Autodesk Inventor part; units mm, degrees
ref_plane "YZ Plane" through (0, 0, 0) normal (1, 0, 0) x (0, 1, 0)
ref_plane "XZ Plane" through (0, 0, 0) normal (0, 1, 0) x (-1, 0, 0)
ref_plane "XY Plane" through (0, 0, 0) normal (0, 0, 1) x (1, 0, 0)
sketch "Sketch1" plane through (0, 0, 0) normal (0, 1, 0) x (-1, 0, 0)
  line L0 (50, 37.5) -> (-50, 37.5)
  line L1 (-50, 37.5) -> (-50, -37.5)
  line L2 (-50, -37.5) -> (50, -37.5)
  line L3 (50, -37.5) -> (50, 37.5)
  line L4 (50, 37.5) -> (-50, -37.5) construction
  line L5 (-50, 37.5) -> (50, -37.5) construction
  line L6 (0, 0) -> (-10, 0)
  line L7 (-10, 0) -> (-10, 8)
  line L8 (-10, 0) -> (-2, 0) construction
  line L9 (-10, 0) -> (-10, -8)
  line L10 (-10, 0) -> (-2, 0) construction
  line L11 (-10, 8) -> (-43, 8) construction
  line L12 (-10, 9.6) -> (-43, 9.6)
  line L13 (-43, 6.4) -> (-10, 6.4)
  arc A0 (-10, 6.4) -> (-10, 9.6) centre (-10, 8) ccw
  arc A1 (-43, 9.6) -> (-43, 6.4) centre (-43, 8) ccw
  line L14 (-10, 8) -> (23, 8) construction
  line L15 (0, 0) -> (-50, 0)
  line L16 (-10, -8) -> (-43, -8) construction
  line L17 (-10, -6.4) -> (-43, -6.4)
  line L18 (-43, -9.6) -> (-10, -9.6)
  arc A2 (-10, -9.6) -> (-10, -6.4) centre (-10, -8) ccw
  arc A3 (-43, -6.4) -> (-43, -9.6) centre (-43, -8) ccw
  line L19 (-10, -8) -> (23, -8) construction
  line L20 (0, 37.5) -> (0, -37.5)
  line L21 (10, 0) -> (10, 8)
  line L22 (10, 0) -> (10, -8)
  line L23 (10, 8) -> (43, 8) construction
  line L24 (10, 9.6) -> (43, 9.6)
  line L25 (43, 6.4) -> (10, 6.4)
  arc A4 (10, 9.6) -> (10, 6.4) centre (10, 8) ccw
  arc A5 (43, 6.4) -> (43, 9.6) centre (43, 8) ccw
  line L26 (10, -8) -> (43, -8) construction
  line L27 (10, -6.4) -> (43, -6.4)
  line L28 (43, -9.6) -> (10, -9.6)
  arc A6 (10, -6.4) -> (10, -9.6) centre (10, -8) ccw
  arc A7 (43, -9.6) -> (43, -6.4) centre (43, -8) ccw
  point P0 (-26.5, 8)
  point P1 (-26.5, -8)
  point P2 (26.5, 8)
  point P3 (26.5, -8)
  dimension "d0" = 100
  dimension "d1" = 75
  dimension "d2" = 10
  dimension "d3" = 8
  dimension "d4" = 90
  dimension "d5" = 8
  dimension "d6" = 90
  dimension "d7" = 33
  dimension "d8" = 180
  dimension "d9" = 3.2
  dimension "d10" = 33
  dimension "d11" = 180
  dimension "d12" = 3.2
extrude "Extrusion1" add sketch "Sketch1" along normal blind 10
sketch "Sketch2" plane through (0, 10, 0) normal (0, 1, 0) x (1, 0, 0)
  line L0 (50, 37.5) -> (-50, 37.5)
  line L1 (-50, 37.5) -> (50, 37.5)
  line L2 (50, 37.5) -> (50, 84.5)
  line L3 (50, 84.5) -> (-50, 84.5)
  line L4 (-50, 84.5) -> (-50, 37.5)
  point P0 (0, 0)
  dimension "d15" = 47
extrude "Extrusion2" add sketch "Sketch2" against normal blind 10
sketch "Sketch3" plane through (0, 10, 0) normal (0, 1, 0) x (1, 0, 0)
  line L0 (38.0429, 35.7373) -> (1.3429, 35.7373)
  line L1 (1.3429, 35.7373) -> (1.3429, 72.4373)
  line L2 (1.3429, 72.4373) -> (38.0429, 72.4373)
  line L3 (38.0429, 72.4373) -> (38.0429, 35.7373)
  circle A0 centre (1.3429, 72.4373) radius 1.65
  circle A1 centre (1.3429, 35.7373) radius 1.65
  circle A2 centre (38.0429, 35.7373) radius 1.65
  circle A3 centre (38.0429, 72.4373) radius 1.65
  line L4 (-28.9751, 35.7373) -> (-28.9751, 72.4373)
  circle A4 centre (-28.9751, 72.4373) radius 1.65
  circle A5 centre (-28.9751, 35.7373) radius 1.65
  point P0 (0, 0)
  dimension "d18" = 36.7
  dimension "d19" = 36.7
  dimension "d20" = 3.3
  dimension "d21" = 3.3
  dimension "d22" = 3.3
  dimension "d23" = 3.3
  dimension "d24" = 36.7
  dimension "d25" = 3.3
  dimension "d26" = 3.3
extrude "Extrusion3" cut sketch "Sketch3" against normal blind 10 contours A1 L1 L0 | L0 L1 A1 | A2 L3 L0 | L0 L3 A2 | A0 L2 L1 | L1 L2 A0 | A3 L2 L3 | L3 L2 A3 | A4 | A5
sketch "Sketch4" plane through (0, 10, 0) normal (0, 1, 0) x (1, 0, 0)
  point P0 (0, 0)
fillet "Fillet1" radius 7 4 edges at (-50, 5, 37.5) (50, 5, 37.5) (50, 5, -84.5) (-50, 5, -84.5)
properties part number "bas" material "Polycarbonate, Clear"
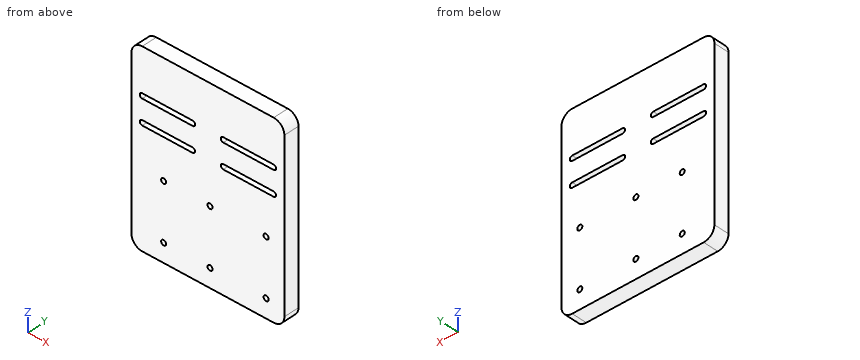
The listing builds one solid part. Answer for the finished solid, in the listing's coordinates (mm). Coordinates: 2 decimals unless noted, no trailing zeros. Loops run counter-clockwise (first coordinate to the right, second up) from the corner with the lowest first, then second, coordinate; pieces in that order, holes last. Notation, with made-up numbers: (-14.75, 0.25) - (36.25, 0.25) arc R24 cw to (36.25, 18.25) - close; hole circle Ø1 at (-32, -32). An arc over 180 degrees is marked (long way). Use a Markdown table: item, result. Add a question column.
1) The part is cut by section C-C, the plane y = 4. State how many separate pieces and enclosed holes the cut face has, and give its area (3 significant figures).
2) The part is cut by section B-B, the plane z = 8. Give the vertices of the cut face in (x, y).
3) Find the intervals of material crossed by line 1 (Z direction, x = -13, y = 5.75); line 2 (Z direction, x = -29, y = 8.75); line 3 (X direction, y = 4.25, z = -73.5), in increasing order.
4) The part is cut by section A-A, the plane x = -21. Give the vertices of the cut face in (y, z).
Here are the results:
| question | item | result |
|---|---|---|
| 1 | separate pieces | 1 |
| 1 | enclosed holes | 10 |
| 1 | area | 11,700 mm^2 |
| 2 | outline | (-50, 0) - (-44.6, 0) - (-44.6, 10) - (-50, 10) - close; (-8.4, 0) - (8.4, 0) - (8.4, 10) - (-8.4, 10) - close; (44.6, 0) - (50, 0) - (50, 10) - (44.6, 10) - close |
| 3 | line 1 | z = -84.5 to -9.6, -6.4 to 6.4, 9.6 to 37.5 |
| 3 | line 2 | z = -84.5 to -74.09, -70.79 to -37.39, -34.09 to -9.6, -6.4 to 6.4, 9.6 to 37.5 |
| 3 | line 3 | x = -50 to -30.24, -27.71 to 0.08, 2.61 to 36.78, 39.31 to 50 |
| 4 | outline | (0, -84.5) - (10, -84.5) - (10, -9.6) - (0, -9.6) - close; (0, -6.4) - (10, -6.4) - (10, 6.4) - (0, 6.4) - close; (0, 9.6) - (10, 9.6) - (10, 37.5) - (0, 37.5) - close |
